Solid Edge part; units mm, degrees
sketch "Sketch1" plane through (0.0007, 14.651, 5) normal (0, 0, 1) x (1, 0, 0)
  line L0 (-114.0407, 98.8093) -> (-57.2599, 131.5929)
  arc A0 (-54.1474, 131.5247) -> (-57.2599, 131.5929) centre (-55.7598, 128.9948) ccw
  arc A1 (-47.0142, 137.1861) -> (-48.7662, 134.4664) centre (-45.7662, 134.458) ccw
  arc A2 (-47.0142, 137.1861) -> (-26.9146, 142.5706) centre (-21.0226, 80.3698) cw
  arc A3 (-24.0376, 141.0909) -> (-26.9146, 142.5706) centre (-26.6317, 139.5839) ccw
  arc A4 (-15.245, 142.849) -> (-17.9063, 141.2336) centre (-15.245, 139.849) ccw
  line L1 (-15.245, 142.849) -> (15.2436, 142.849)
  arc A5 (17.905, 141.2336) -> (15.2436, 142.849) centre (15.2436, 139.849) ccw
  arc A6 (26.9132, 142.5696) -> (24.036, 141.0904) centre (26.6298, 139.583) ccw
  arc A7 (26.9132, 142.5696) -> (47.0027, 137.1869) centre (21.0099, 80.3561) cw
  arc A8 (48.7549, 134.4673) -> (47.0027, 137.1869) centre (45.7549, 134.4587) ccw
  arc A9 (57.2487, 131.5943) -> (54.1362, 131.526) centre (55.7487, 128.9962) ccw
  line L2 (57.2487, 131.5943) -> (114.0299, 98.8129)
  arc A10 (115.5271, 96.0833) -> (114.0299, 98.8129) centre (112.5299, 96.2148) ccw
  arc A11 (124.0003, 92.7805) -> (120.7849, 92.9052) centre (122.2944, 90.3127) ccw
  arc A12 (124.0003, 92.7805) -> (155.0355, 39.027) centre (82.7747, 33.1424) cw
  arc A13 (153.5358, 36.1799) -> (155.0355, 39.027) centre (152.0454, 38.7835) ccw
  arc A14 (155.2747, 27.3761) -> (153.6593, 30.0375) centre (152.2747, 27.3761) ccw
  line L3 (155.2747, 27.3761) -> (155.2747, -38.192)
  arc A15 (153.6593, -40.8534) -> (155.2747, -38.192) centre (152.2747, -38.192) ccw
  arc A16 (154.9954, -49.8615) -> (153.5161, -46.9844) centre (152.0088, -49.5782) ccw
  arc A17 (154.9954, -49.8615) -> (149.6134, -69.9554) centre (92.7533, -43.9583) cw
  arc A18 (146.8942, -71.7079) -> (149.6134, -69.9554) centre (146.8851, -68.7079) ccw
  arc A19 (144.0217, -80.2016) -> (143.9534, -77.0892) centre (141.4236, -78.7016) ccw
  line L4 (144.0217, -80.2016) -> (127.6444, -108.5679)
  arc A20 (122.7007, -116.5716) -> (122.8583, -113.3403) centre (120.256, -114.8329) ccw
  arc A21 (77.6703, -142.5696) -> (122.7007, -116.5716) centre (71.767, -80.3476) ccw
  arc A22 (74.7931, -141.0904) -> (77.6703, -142.5696) centre (77.3869, -139.583) ccw
  arc A23 (66.0007, -142.849) -> (68.6621, -141.2336) centre (66.0007, -139.849) ccw
  line L5 (5.7656, -142.849) -> (66.0007, -142.849)
  arc A24 (3.1042, -141.2336) -> (5.7656, -142.849) centre (5.7656, -139.849) ccw
  arc A25 (-5.767, -142.849) -> (-3.1056, -141.2336) centre (-5.767, -139.849) ccw
  line L6 (-66.0021, -142.849) -> (-5.767, -142.849)
  arc A26 (-68.6634, -141.2336) -> (-66.0021, -142.849) centre (-66.0021, -139.849) ccw
  arc A27 (-77.6716, -142.5694) -> (-74.7944, -141.0903) centre (-77.3881, -139.5828) ccw
  arc A28 (-122.6994, -116.5717) -> (-77.6716, -142.5694) centre (-71.7665, -80.349) ccw
  arc A29 (-122.857, -113.3404) -> (-122.6994, -116.5717) centre (-120.2547, -114.833) ccw
  arc A30 (-128.7762, -106.6053) -> (-126.0465, -108.1024) centre (-126.1781, -105.1053) ccw
  line L7 (-144.0218, -80.199) -> (-128.7762, -106.6053)
  arc A31 (-143.9535, -77.0865) -> (-144.0218, -80.199) centre (-141.4237, -78.699) ccw
  arc A32 (-149.6144, -69.9531) -> (-146.8949, -71.7053) centre (-146.8862, -68.7053) ccw
  arc A33 (-154.9987, -49.8585) -> (-149.6144, -69.9531) centre (-92.7672, -43.9523) ccw
  arc A34 (-153.5196, -46.9813) -> (-154.9987, -49.8585) centre (-152.0122, -49.5751) ccw
  arc A35 (-155.2786, -38.189) -> (-153.6631, -40.8503) centre (-152.2786, -38.1889) ccw
  line L8 (-155.2818, 27.3758) -> (-155.2786, -38.189)
  arc A36 (-153.6665, 30.0373) -> (-155.2818, 27.3758) centre (-152.2818, 27.376) ccw
  arc A37 (-155.0428, 39.0267) -> (-153.5432, 36.1796) centre (-152.0527, 38.7832) ccw
  arc A38 (-124.0109, 92.7765) -> (-155.0428, 39.0267) centre (-82.7847, 33.1421) ccw
  arc A39 (-120.7955, 92.9014) -> (-124.0109, 92.7765) centre (-122.3049, 90.3088) ccw
  arc A40 (-114.0407, 98.8093) -> (-115.5378, 96.0796) centre (-112.5406, 96.2112) ccw
  arc A41 (-48.7662, 134.4664) -> (-54.1474, 131.5247) centre (-52.2662, 134.4761) cw
  arc A42 (-17.9064, 141.2336) -> (-24.0377, 141.0909) centre (-21.0113, 142.849) cw
  arc A43 (24.036, 141.0904) -> (17.905, 141.2336) centre (21.0099, 142.849) cw
  arc A44 (54.1362, 131.526) -> (48.7549, 134.4673) centre (52.2549, 134.4774) cw
  arc A45 (120.7849, 92.9052) -> (115.5271, 96.0832) centre (119.0237, 95.9298) cw
  arc A46 (153.6593, 30.0375) -> (153.5358, 36.1799) centre (155.2747, 33.1424) cw
  arc A47 (153.5161, -46.9844) -> (153.6593, -40.8534) centre (155.2747, -43.9583) cw
  arc A48 (143.9534, -77.0891) -> (146.8942, -71.7079) centre (146.9048, -75.2079) cw
  arc A49 (122.8584, -113.3404) -> (127.6444, -108.5679) centre (125.8944, -111.599) cw
  arc A50 (68.6621, -141.2336) -> (74.7931, -141.0904) centre (71.767, -142.849) cw
  arc A51 (-3.1056, -141.2336) -> (3.1042, -141.2336) centre (-0.0007, -142.849) cw
  arc A52 (-74.7944, -141.0903) -> (-68.6635, -141.2336) centre (-71.7684, -142.849) cw
  arc A53 (-126.0466, -108.1024) -> (-122.857, -113.3404) centre (-125.8931, -111.599) cw
  arc A54 (-146.8949, -71.7053) -> (-143.9536, -77.0866) centre (-146.905, -75.2053) cw
  arc A55 (-153.6632, -40.8503) -> (-153.5196, -46.9813) centre (-155.2784, -43.9553) cw
  arc A56 (-153.5432, 36.1796) -> (-153.6665, 30.0373) centre (-155.2821, 33.1421) cw
  arc A57 (-115.5377, 96.0796) -> (-120.7955, 92.9014) centre (-119.0344, 95.926) cw
  line L9 (-56.0166, 140.971) -> (-122.7845, 102.4212)
  arc A58 (-162.7821, 33.1421) -> (-122.7845, 102.4212) centre (-82.7847, 33.1421) cw
  line L10 (-162.7821, 33.1421) -> (-162.7784, -43.9553)
  arc A59 (-162.7784, -43.9553) -> (-153.4002, -78.9553) centre (-92.7784, -43.9553) ccw
  line L11 (-132.3882, -115.349) -> (-153.4002, -78.9553)
  arc A60 (-132.3882, -115.349) -> (-71.7683, -150.349) centre (-71.7665, -80.349) ccw
  line L12 (71.767, -150.349) -> (-71.7683, -150.349)
  arc A61 (71.767, -150.349) -> (132.3896, -115.349) centre (71.7678, -80.349) ccw
  line L13 (132.3896, -115.349) -> (153.4002, -78.9576)
  arc A62 (162.7747, -43.9583) -> (153.4002, -78.9576) centre (92.791, -43.9684) cw
  line L14 (162.7747, 33.1424) -> (162.7747, -43.9583)
  arc A63 (122.7736, 102.4251) -> (162.7747, 33.1424) centre (82.7747, 33.1424) cw
  line L15 (56.0045, 140.9728) -> (122.7736, 102.4251)
  arc A64 (21.0099, 150.349) -> (56.0045, 140.9728) centre (21.008, 80.349) cw
  line L16 (-21.0112, 150.349) -> (21.0099, 150.349)
  arc A65 (-32.5074, 149.4015) -> (-21.0112, 150.349) centre (-20.997, 79.961) cw
  arc A66 (-44.641, 146.2432) -> (-32.5074, 149.4015) centre (-21.0122, 80.3518) cw
  arc A67 (-56.0166, 140.971) -> (-44.641, 146.2432) centre (-21.0122, 80.3518) cw
  circle A68 centre (-71.7683, -142.849) radius 1.5
  circle A69 centre (-0.0007, -142.849) radius 1.5
  circle A70 centre (-125.893, -111.599) radius 1.5
  circle A71 centre (-146.905, -75.2053) radius 1.5
  circle A72 centre (-155.2784, -43.9553) radius 1.5
  circle A73 centre (-155.2821, 33.1421) radius 1.5
  circle A74 centre (-119.0344, 95.9261) radius 1.5
  circle A75 centre (-52.2662, 134.4761) radius 1.5
  circle A76 centre (-21.0112, 142.849) radius 1.5
  circle A77 centre (21.0099, 142.849) radius 1.5
  circle A78 centre (52.2549, 134.4774) radius 1.5
  circle A79 centre (119.0237, 95.9298) radius 1.5
  circle A80 centre (155.2747, 33.1424) radius 1.5
  circle A81 centre (155.2747, -43.9583) radius 1.5
  circle A82 centre (146.9048, -75.2079) radius 1.5
  circle A83 centre (125.8944, -111.599) radius 1.5
  circle A84 centre (71.767, -142.849) radius 1.5
extrude "ExtrudedProtrusion_7" add sketch "Sketch1" along normal blind 5
sketch "Sketch2" plane through (-0.003, 14.651, 10) normal (0, 0, 1) x (1, 0, 0)
  line L0 (-170.0115, -5.4066) -> (169.0999, -5.4066)
  line L1 (169.0999, -5.4066) -> (169.0999, -159.984)
  line L2 (169.0999, -159.984) -> (-170.0115, -159.984)
  line L3 (-170.0115, -159.984) -> (-170.0115, -5.4066)
extrude "Cutout1" cut sketch "Sketch2" against normal up to next
sketch "Sketch3" plane through (-0.003, 87.1222, 10) normal (0, 0, 1) x (0.866, -0.5, 0)
  line L0 (-38.9352, 67.4463) -> (43.5625, -75.4492)
  line L1 (43.5625, -75.4492) -> (205.1735, 17.8535)
  line L2 (205.1735, 17.8535) -> (122.2113, 161.5535)
  line L3 (122.2113, 161.5535) -> (-38.8416, 68.573)
  line L4 (-38.9352, 67.4463) -> (-38.8416, 68.573)
extrude "Cutout2" cut sketch "Sketch3" against normal up to next
properties material "Polycarbonate"
Geometry: final body of the model. Coordinates: model frame, mm. A direction names the side the tool comes from. Round coordinates to 2 decimals unless told otherwise and drop trailing zeros. Write each loop counter-clockwise with the first axis right and the second up, starting at its lowest first coordinate (ties: lowest second). Pieces come first, ordered by that corner, then holes. Notation, with made-up numbers: (79, -21.75) -> (102, -21.75) arc R16 cw to (102, 2.25) -> close; hole circle Ø5 at (-13.5, 77.5). An arc over 180 degrees is marked (long way). Use CSV: the item, a comma, the result in double quotes. Start each with the question number.
Q1. First-contact query: pin 1 Ø2 at (x, z) = (-62.5, 8.5) entering from -Y; pin 2 Ø1.8 at (x, y) = (-155.28, 47.79) entering from -Z; pin 3 Ø2.5 at (y, z) = (19.5, 8.5) entering from +X; pin 4 Ø1.5 at (x, z) = (-7.5, 7.5) entering from -Y. Flat tips, straight axial feed; report the tip coordinate or a pass-through.
Q2. Pull-direction query (X, two-part tool) for faces 1 (the face through (-11, 165, 7)), 2 (the face through (-37.331, 155.334, 7.465)), 3 (the face through (-151.78, 47.78, 7.46)), 4 (the face through (-21, 154, 7)); classes: pulls with the +X half, pulls with the -X half, needs draft (parallel to the pull), parting line crosses it, or undercut.
Q3. Section C-C (y = 97.5). Return loops of the section in (x, z).
Q4. Section A-A (z = 6.85). Give the number of separate pieces and of enclosed holes in the cut face, plus the area to 3 significant figures.
Q5. Reachability of faces 5 (the face through (-112, 116, 10)), 6 (the face through (-8, 157.5, 7)) from +Z, -Z, +X, -X, +Y, -Y: full face, straight path, thin tool, end or side. Return the list, or none.
Q6. Line query: L1, parallel to X at y = 37, z = 6.3; L2, parallel to Y at x = -11, z = 9.05; L3, parallel to X at y = 150, z = 5.65. Output: solid intervals per line, ascending.
Q7. Section B-B (x = -13). Return loops of the section in (y, z).
Result sheet:
1,pin 1,"y = 142.64"
1,pin 2,"through"
1,pin 3,"x = -155.28"
1,pin 4,"y = 157.5"
2,face 1,"needs draft"
2,face 2,"undercut"
2,face 3,"pulls with the +X half"
2,face 4,"undercut"
3,outline,"(-145.46, 5) -> (-135.56, 5) -> (-135.56, 10) -> (-145.46, 10) -> close"
4,separate pieces,"1"
4,enclosed holes,"4"
4,area,"1,940 mm²"
5,face 5,"+Z, +X, -X, +Y, -Y"
5,face 6,"+Z, -Z, +X, -Y"
6,L1,"-162.78 to -155.28"
6,L2,"157.5 to 165"
6,L3,"-65.75 to -53.49, -51.05 to -48.63"
7,outline,"(157.5, 5) -> (165, 5) -> (165, 10) -> (157.5, 10) -> close"
